The model under review builds one solid part; all positions refer to its coordinate system, in mm. Face numbers are marked on the shaded views. A direction names the side the tool comes from. Coordinates: 2 decimals unless noted, no trailing zeros. Order: outer loops, then holes, each group sorted by start corner. A loop starts at its lowest first (then second) coordinate and runs counter-clockwise, first axis right, second up. Notation, with made-up numbers: (4, 21) -> (15, 21) arc R7 cw to (15, 30) -> close; hole circle Ø11 at (25, -11.5). An arc over 180 degrees is marked (long way). Use one line per item in the form item = value.
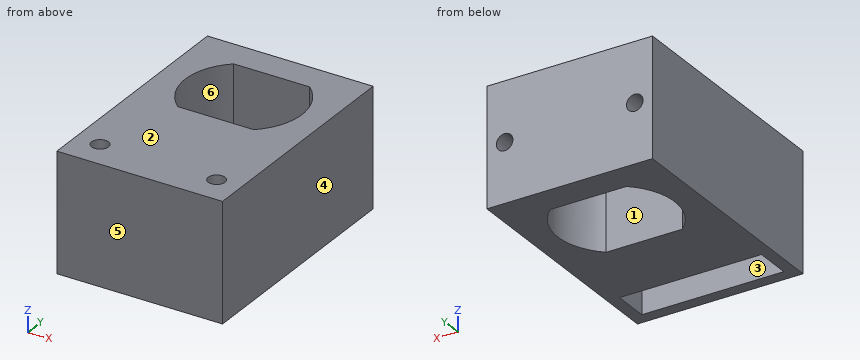
from build123d import *

# Parameters (mm, degrees)
SKETCH4_W           = 28
SKETCH4_H           = 40.4
BOSS_EXTRUDE1_DEPTH = 20
CUT_EXTRUDE1_DEPTH  = 21
SKETCH6_R           = 1.42
CUT_EXTRUDE3_DEPTH  = 10
SKETCH7_W           = 24
SKETCH7_H           = 6
CUT_EXTRUDE4_DEPTH  = 10
SKETCH8_R           = 1.4
CUT_EXTRUDE5_DEPTH  = 8


with BuildPart() as part:
    # Sketch4 → Boss-Extrude1 (new body)
    with BuildSketch(Plane.XY):
        Rectangle(SKETCH4_W, SKETCH4_H)
    extrude(amount=BOSS_EXTRUDE1_DEPTH)

    # Sketch5 → Cut-Extrude1 (cut, through all)
    with BuildSketch(Plane.XY.offset(20)):
        with BuildLine():
            Line((-6.423832579, 15.2), (6.423832579, 15.2))
            ThreePointArc((6.423832579, 15.2), (9.875, 7.7), (6.423832579, 0.2))
            Line((6.423832579, 0.2), (-6.423832579, 0.2))
            ThreePointArc((-6.423832579, 0.2), (-9.875, 7.7), (-6.423832579, 15.2))
        make_face()
    extrude(amount=-CUT_EXTRUDE1_DEPTH, mode=Mode.SUBTRACT)

    # Sketch6 → Cut-Extrude3 (cut)
    with BuildSketch(Plane.XY.offset(20)):
        with Locations((-9.85, -15.2)):
            Circle(SKETCH6_R)
        with Locations((9.85, -15.2)):
            Circle(SKETCH6_R)
    extrude(amount=-CUT_EXTRUDE3_DEPTH, mode=Mode.SUBTRACT)

    # Sketch7 → Cut-Extrude4 (cut)
    with BuildSketch(Plane.XY):
        with Locations((0, -15.2)):
            Rectangle(SKETCH7_W, SKETCH7_H)
    extrude(amount=CUT_EXTRUDE4_DEPTH, mode=Mode.SUBTRACT)

    # Sketch8 → Cut-Extrude5 (cut)
    with BuildSketch(Plane(origin=(0, 20.2, 0), x_dir=(1, 0, 0), z_dir=(0, 1, 0))):
        with Locations((-11, -10)):
            Circle(SKETCH8_R)
        with Locations((11, -10)):
            Circle(SKETCH8_R)
    extrude(amount=-CUT_EXTRUDE5_DEPTH, mode=Mode.SUBTRACT)


solid = part.part
Item 1: To check wall thickness, follow L1, parallel to X at y = 17.25, z = 10; L2, parallel to Y at x = -0.5, z = 6; L3, parallel to Y at x = 10.75, z = 6.5. State the ranges of each line that lie inside material, in increasing order. Write a range as from..to.
Results found:
L1 = -14..-12.4, -9.6..9.6, 12.4..14
L2 = -20.2..-18.2, -12.2..0.2, 15.2..20.2
L3 = -20.2..-18.2, -12.2..20.2
Item 2: We need section D-D (y = 16). Write out the cut boundary in (x, z).
Results found:
outline = (-14, 0) -> (14, 0) -> (14, 20) -> (-14, 20) -> close; hole circle Ø2.8 at (-11, 10); hole circle Ø2.8 at (11, 10)
Item 3: We need section C-C (x = 2.75). Write out the cut boundary in (y, z), plus the area to 3 significant figures.
Results found:
outline = (-20.2, 0) -> (-18.2, 0) -> (-18.2, 10) -> (-12.2, 10) -> (-12.2, 0) -> (0.2, 0) -> (0.2, 20) -> (-20.2, 20) -> close; (15.2, 0) -> (20.2, 0) -> (20.2, 20) -> (15.2, 20) -> close
area = 448 mm²
Item 4: Clearance check with flat-ended pins moving along their axes: pin 1 (0.8 mm diameter, centred on x = -11.5, z = 10, fed in from +Y); pin 2 (2.5 mm diameter, centred on x = 9.85, y = -15.2, fed in from -Z); pin 3 (5 mm diameter, centred on x = 8, y = -15.5, fed in from -Z). State where each tip first meets the part, or that it passes through.
Results found:
pin_1 = 12.2
pin_2 = through
pin_3 = 10
Item 5: We need section A-A (y = -15.2). Write out the cut boundary in (x, z), plus the area to 3 significant figures.
Results found:
outline = (-14, 0) -> (-12, 0) -> (-12, 10) -> (-11.27, 10) -> (-11.27, 20) -> (-14, 20) -> close; (-8.43, 10) -> (8.43, 10) -> (8.43, 20) -> (-8.43, 20) -> close; (11.27, 10) -> (12, 10) -> (12, 0) -> (14, 0) -> (14, 20) -> (11.27, 20) -> close
area = 263 mm²
Item 6: We need section B-B (z = 3). Write out the cut boundary in (x, y) (3 decimals), plus the area to 3 significant figures.
Results found:
outline = (-14, -20.2) -> (14, -20.2) -> (14, 20.2) -> (-14, 20.2) -> close; hole (-12, -18.2) -> (12, -18.2) -> (12, -12.2) -> (-12, -12.2) -> close; hole (-6.424, 0.2) -> (6.424, 0.2) arc R9.875 ccw to (6.424, 15.2) -> (-6.424, 15.2) arc R9.875 ccw to start
area = 723 mm²
Item 7: Tool access review of the marked faces 1, 2 and 3: name each direction out of +Z, -Z, +X, -X, +Y, -Y from which nothing blocks a thin tool from reaching the whole face with its end or side.
Results found:
face_1 = +Z, -Z
face_2 = +Z, +X, -X, +Y, -Y
face_3 = -Z
Item 8: Draft analysis for pull direction Y (two halves, no side actions). For the marked faces 4, 5 and 6, state which applies: released by +Y, released by -Y, zero draft, split by the parting line, or undercut.
Results found:
face_4 = zero draft
face_5 = released by -Y
face_6 = undercut
